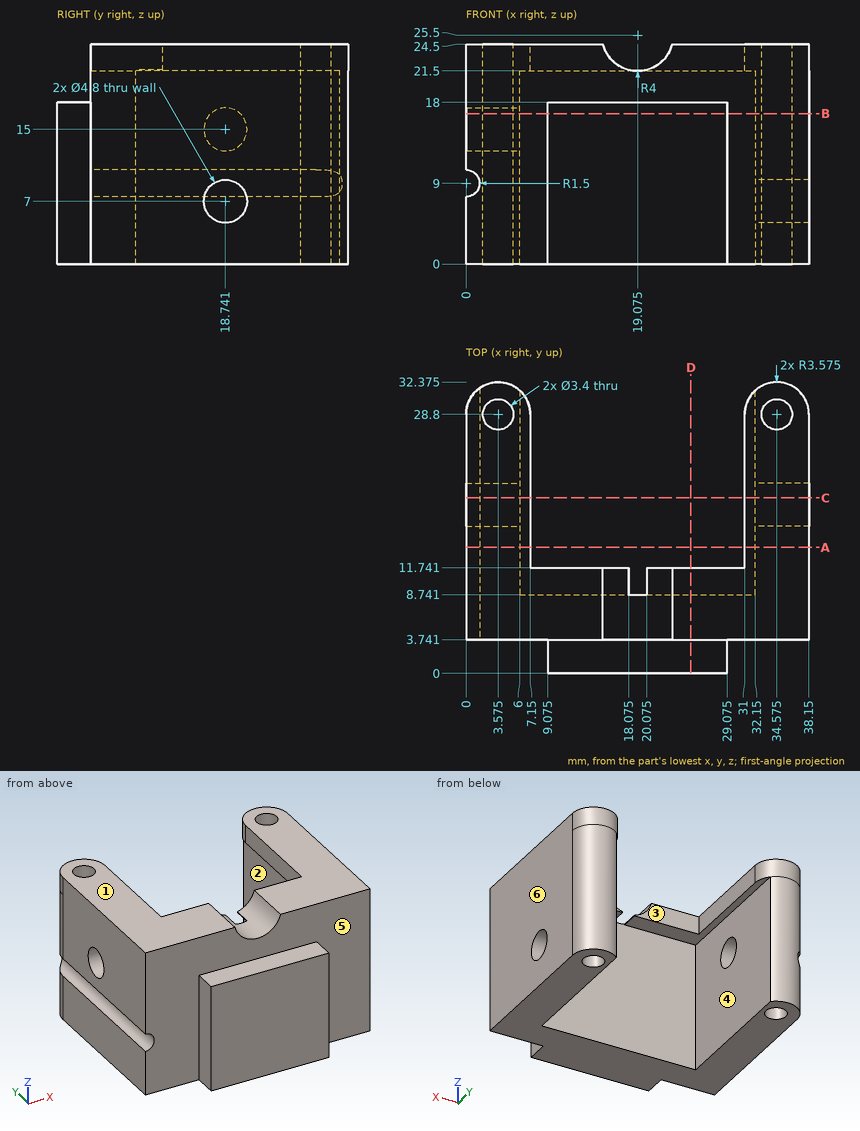
Could you check a few things on this drawing? It's one solid part, dimensions in mm from its lowest x, y, z. A direction names the side the tool comes from. Give positions to 0.01 mm unless a question says otherwise; leave off trailing zeros. Order: outer loops, then holes, each group sorted by start corner. A loop starts at its lowest first (then second) coordinate and runs counter-clockwise, first axis right, second up. Notation, with made-up numbers: (-8.5, 34.5) - (-1.5, 34.5) arc R31 cw to (-1.5, 70.5) - close; hole circle Ø7 at (64, -24). An arc over 180 degrees is marked (long way). Answer as a JSON object with one key per item and string values. Group by question number.
Item 1: If we section it at B-B on z = 16.75: Give the number of separate pieces and of enclosed holes in the cut face, and give its area (3 significant figures).
Item 2: Please list where these lines run through material, in increasing order: probe 1 along X at (y, z) = (28.8, 15) (3 decimals); probe 2 along X at (y, z) = (15.5, 5); probe 3 along Y at (x, z) = (2.4, 15).
Item 3: Which directions (+Z, -Z, +X, -X, +Y, -Y) give clear straight access to the entire face, cutting with the end or side of a thin tool? Please do the marked faces 1, 2 and 3.
Item 4: If we section it at C-C on y = 19.5: Please give me the cut outline in (x, z), and give its area (3 significant figures).
Item 5: If we section it at A-A on y = 14: Please give me the cut outline in (x, z), and give its area (3 significant figures).
Item 6: For P1, Ø4, axis at x = 8.5, y = 15.5, coming from the -Z side; P2, Ø2.5, axis at x = 26, z = 23.5, coming from the +Y side; P3, Ø5.5, axis at y = 18.74, z = 7, coming from the +X side; P4, Ø6.5, axis at x = 17, z = 6.5, coming from the +Y side, each with a flat end and sliding along its axis, tell me the tip position at first contact or that it passes through.
Item 7: If we mould it in two halves opening along X, with no side actions, what happens to the marked faces 4, 5 and 6? For each: pulls with the +X half, pulls with the -X half, needs draft (parallel to the pull), parting line crosses it, or undercut.
Item 8: If we section it at D-D on x = 25: Please give me the cut outline in (y, z), and give its area (3 significant figures).
Result set:
{
 "1": {"separate pieces": "2", "enclosed holes": "2", "area": "504 mm²"},
 "2": {"probe 1": "0 to 1.875, 5.275 to 6, 32.15 to 32.875, 36.275 to 38.15", "probe 2": "0 to 6, 32.15 to 38.15", "probe 3": "3.74 to 16.34, 21.14 to 27.57, 30.03 to 32.18"},
 "3": {"face 1": "+Z, +X, -X, +Y, -Y", "face 2": "-Z, +Y", "face 3": "+Z, -Z, +Y"},
 "4": {"outline": "(0, 0) - (6, 0) - (6, 12.72) - (0, 12.72) - (0, 10.5) arc R1.5 cw to (0, 7.5) - close; (0, 17.28) - (6, 17.28) - (6, 21.5) - (7.15, 21.5) - (7.15, 24.5) - (0, 24.5) - close; (31, 21.5) - (32.15, 21.5) - (32.15, 9.28) - (38.15, 9.28) - (38.15, 24.5) - (31, 24.5) - close; (32.15, 0) - (38.15, 0) - (38.15, 4.72) - (32.15, 4.72) - close", "area": "243 mm²"},
 "5": {"outline": "(0, 0) - (6, 0) - (6, 21.5) - (7.15, 21.5) - (7.15, 24.5) - (0, 24.5) - (0, 10.5) arc R1.5 cw to (0, 7.5) - close; (31, 21.5) - (32.15, 21.5) - (32.15, 0) - (38.15, 0) - (38.15, 24.5) - (31, 24.5) - close", "area": "297 mm²"},
 "6": {"P1": "z = 21.5", "P2": "y = 11.74", "P3": "x = 38.15", "P4": "y = 8.74"},
 "7": {"face 4": "undercut", "face 5": "needs draft", "face 6": "pulls with the +X half"},
 "8": {"outline": "(0, 0) - (8.74, 0) - (8.74, 21.5) - (11.74, 21.5) - (11.74, 24.5) - (3.74, 24.5) - (3.74, 18) - (0, 18) - close", "area": "199 mm²"}
}
